Part print with two shaded views. Sizes in mm from the minimum x, y, z corner. A direction names the side the tool comes from. Round coordinates to 2 decimals unless told otherwise and drop trailing zeros. Write each loop counter-clockwise with the first axis right and the second up, starting at its lowest first coordinate (ties: lowest second). Pieces come first, ordered by that corner, then holes. Notation, with made-up numbers: M 59.25,-17 L 96.25,-17 A12 cw 96.25,-12 Z; hole C 28,62 d6. An arc over 180 degrees is marked long. Use one line per item in the form item = value. Start each with the question number.
Item 1: Probe L1, parallel to Y at x = 8.5, z = 3.25; L2, parallel to Y at x = 4.75, z = 4.5; L3, parallel to X at y = 26.5, z = 3.5 (1 decimal). List the from-to ranges inside material, lowest first.
Item 2: Which spindle directions (+Z, -Z, +X, -X, +Y, -Y) get a long thin tool onto all of the face, cutting with end or side? Do the marked faces 1, 2 and 3. Say none if no direction does.
Item 3: Flat gauge pins, fed straight in: pin 1 Ø0.7 at (y, z) = (26.5, 5.5) entering from +X; pin 2 Ø1 at (x, y) = (7, 26) entering from -Z; pin 3 Ø2 at (x, z) = (9, 5.5) entering from -Y. Where does each tip first touch, or does it go through?
Item 4: Mould opens along X. For the marked faces 4, 5 and 6 say: +X half, -X half, draft (parallel to the pull), parting line (faces both ways), or undercut.
Item 5: Cut at A-A, the plane z = 5. Give the cut face in (x, y), then the cut area to 3 significant figures.
Item 6: Cut at B-B, the plane y = 3. Give the cut face in (x, z), then the cut area to 3 significant figures.
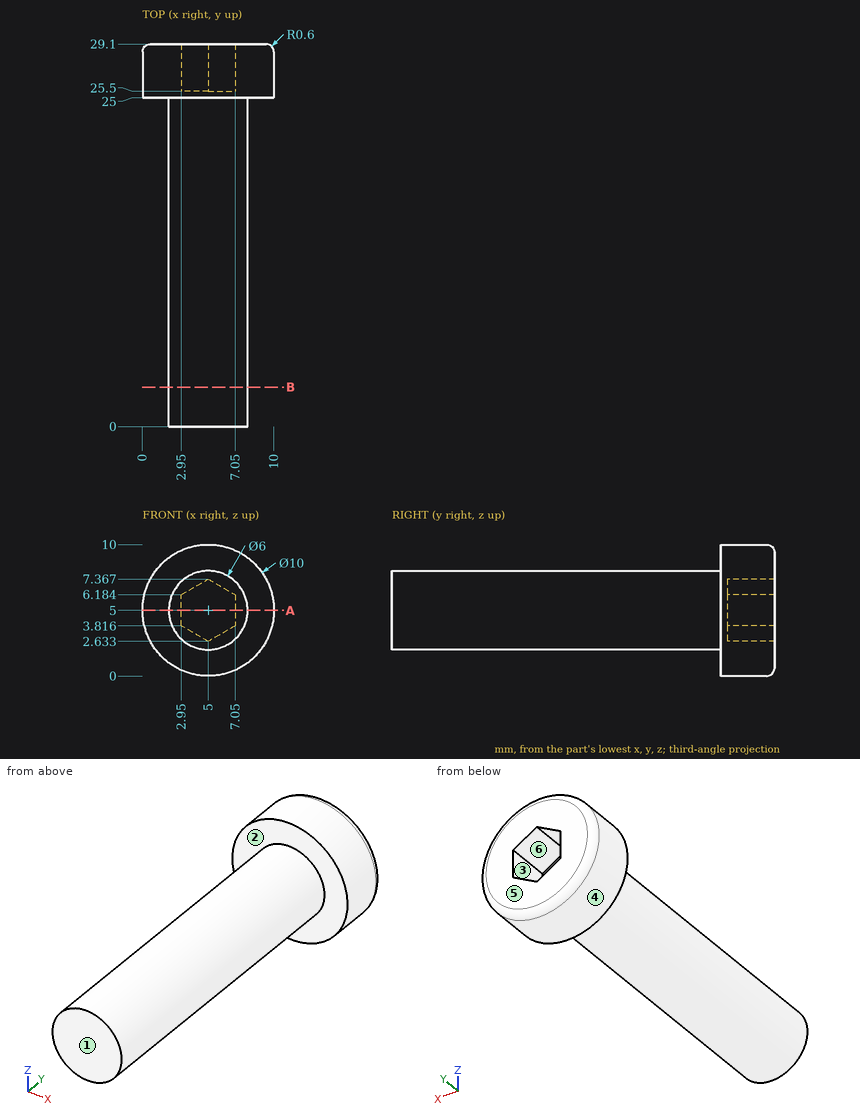
Model answer:
q1.L1 = 25 to 29.1
q1.L2 = 0 to 25.5
q1.L3 = 0.2 to 3.5, 6.5 to 9.8
q2.face_1 = +Z, -Z, +X, -X, -Y
q2.face_2 = -Y
q2.face_3 = +Y
q3.pin_1 = 10
q3.pin_2 = 0.23
q3.pin_3 = 25
q4.face_4 = parting line
q4.face_5 = draft
q4.face_6 = undercut
q5.outline = M 0,25 L 2,25 L 2,0 L 8,0 L 8,25 L 10,25 L 10,28.5 A0.6 ccw 9.4,29.1 L 7.05,29.1 L 7.05,25.5 L 2.95,25.5 L 2.95,29.1 L 0.6,29.1 A0.6 ccw 0,28.5 Z
q5.area = 176 mm²
q6.outline = C 5,5 d6
q6.area = 28.3 mm²
